from build123d import *

# Parameters (mm, degrees)
SKETCH1_R           = 15
BOSS_EXTRUDE1_DEPTH = 100
CHAMFER1_SIZE       = 2
CHAMFER2_SIZE       = 2
CUT_EXTRUDE1_DEPTH  = 60


with BuildPart() as part:
    # Sketch1 → Boss-Extrude1 (new body)
    with BuildSketch(Plane.XY):
        Circle(SKETCH1_R)
    extrude(amount=BOSS_EXTRUDE1_DEPTH)

    # Chamfer1
    chamfer1_edges = [part.edges().sort_by_distance(p)[0] for p in [
        (-15, 0, 100),
    ]]
    chamfer(chamfer1_edges, length=CHAMFER1_SIZE)

    # Chamfer2
    chamfer2_edges = [part.edges().sort_by_distance(p)[0] for p in [
        (-15, 0, 0),
    ]]
    chamfer(chamfer2_edges, length=CHAMFER2_SIZE)

    # Sketch2 → Cut-Extrude1 (cut)
    with BuildSketch(Plane(origin=(0, 0, 0), x_dir=(-1, 0, 0), z_dir=(0, 0, -1))):
        Polygon((-4, 11), (4, 11), (4, 14.456832295), (4, 16.003421776), (-4, 16.003421776), (-4, 14.456832295), align=None)
    extrude(amount=-CUT_EXTRUDE1_DEPTH, mode=Mode.SUBTRACT)


solid = part.part
Geometry: final body of the model. Coordinates: model frame, mm. A direction names the side the tool comes from. Round coordinates to 2 decimals unless told otherwise and drop trailing zeros. Order: outer loops, then holes, each group sorted by start corner. A loop starts at its lowest first (then second) coordinate and runs counter-clockwise, first axis right, second up.
Q1. Mould query, pull axis X, two halves, no side actions, for faces 3 (the face through (-0.54, -13.31, 0.32)), 4 (the face through (0, 0, 0)), 5 (the face through (0, 11, 30)). Classes: released by +X, released by -X, zero draft, split by the parting line, or undercut.
Result sheet:
face 3: split by the parting line
face 4: zero draft
face 5: undercut
Q2. Pin query (flat end, axial travel): pin 1 (3 mm diameter, centred on y = 13, z = 44, fed in from -X); pin 2 (12 mm diameter, centred on y = 1.5, z = 50.5, fed in from -X); pin 3 (2 mm diameter, centred on x = -7.5, z = 22.5, fed in from +Y); pin 4 (4 mm diameter, centred on x = 0, z = 34, fed in from +Y). Return the tip coordinate at first contact, or that it passes through.
Result sheet:
pin 1: stops at x = -9.63
pin 2: stops at x = -15
pin 3: stops at y = 13.52
pin 4: stops at y = 11
Q3. Section A-A, the plane x = 0. Output: boundary loops of the cut face in (y, z).
Result sheet:
outline: (-15, 2) - (-13, 0) - (11, 0) - (11, 60) - (15, 60) - (15, 98) - (13, 100) - (-13, 100) - (-15, 98) - close
Q4. Material intervals for probe 1 along Y at (x, z) = (0, 69); probe 2 along X at (y, z) = (7.5, 77); probe 3 along X at (y, z) = (-0.5, 93.5), sorted ascending.
Result sheet:
probe 1: y = -15 to 15
probe 2: x = -12.99 to 12.99
probe 3: x = -14.99 to 14.99
Q5. Access query for faces 1 (the face through (-3.252, -14.643, 49.328)), 2 (the face through (4, 13, 30)). Directions: +Z, -Z, +X, -X, +Y, -Y. A direction counts if a zero-diameter tool reaches every point of the face in a straight line with its end or side. Return the directions, or none.
Result sheet:
face 1: +Z, -Z
face 2: -Z, +Y
Q6. Section B-B, the plane z = 78.5. Output: boundary loops of the cut face in (x, y).
Result sheet:
outline: circle Ø30 at (0, 0)
